CAD build for the part. Positions are in the model's coordinates, mm. A direction names the side the tool comes from. Round coordinates to 2 decimals unless told otherwise and drop trailing zeros. Order: outer loops, then holes, each group sorted by start corner. A loop starts at its lowest first (then second) coordinate and runs counter-clockwise, first axis right, second up. Notation, with made-up numbers: M 37.5,43 L 61.5,43 A27 ccw 61.5,80 Z; hole C 20,-39.5 d4. An arc over 180 degrees is marked long. Put each result on its own line as item: value.
Autodesk Inventor part; units mm, degrees
ref_plane "YZ Plane" through (0, 0, 0) normal (1, 0, 0) x (0, 1, 0)
ref_plane "XZ Plane" through (0, 0, 0) normal (0, 1, 0) x (-1, 0, 0)
ref_plane "XY Plane" through (0, 0, 0) normal (0, 0, 1) x (1, 0, 0)
sketch "草圖1" plane through (0, 0, 0) normal (0, 0, 1) x (1, 0, 0)
  line L0 (-27.5, 3) -> (27.5, 3) construction
  line L1 (27.5, 3) -> (27.5, 63) construction
  line L2 (27.5, 63) -> (-27.5, 63) construction
  line L3 (-27.5, 63) -> (-27.5, 3) construction
  line L4 (-30.5, 66) -> (30.5, 66)
  line L5 (30.5, 66) -> (30.5, -5.5597)
  line L6 (-30.5, -3) -> (-30.5, 66)
  line L7 (-34.7579, 0) -> (34.7579, 0)
  line L8 (-30.5, -66) -> (30.5, -66)
  line L9 (30.5, -66) -> (30.5, -5.5597)
  line L10 (-30.5, -3) -> (-30.5, -66)
  line L11 (0, 77.5612) -> (0, -87.4517)
  point P0 (0, 3)
  point P1 (0, 3)
  point P2 (0, -3)
  point P3 (0, 0)
  dimension "d0" = 55
  dimension "d1" = 60
  dimension "d2" = 3
  dimension "d3" = 6
extrude "擠出1" add sketch "草圖1" along normal blind 3 and the other way blind 70
shell "薄殼1" thickness 3 removed faces 1 at (-10.1667, 22, -70)
sketch "草圖2" plane through (0, 0, 0) normal (0, 0, 1) x (1, 0, 0)
  line L0 (27.5, 63) -> (27.5, -4)
  line L1 (27.5, -4) -> (-27.5, -4)
  line L2 (-27.5, -4) -> (-27.5, 63)
  line L3 (0, 77.5612) -> (0, -87.4517)
  line L4 (-34.7579, 0) -> (34.7579, 0)
  line L5 (27.5, 63) -> (-27.5, 63)
  point P0 (0, 0)
  point P1 (-27.5, 0)
  point P2 (27.5, 0)
  dimension "d8" = 55
  dimension "d9" = 8
extrude "擠出2" cut sketch "草圖2" along normal blind 3 and the other way blind 2
sketch "草圖3" plane through (0, 0, 0) normal (1, 0, 0) x (0, 1, 0)
  circle A0 centre (59, 0) radius 1.25
  line L0 (-66, 3) -> (66, 3)
  line L1 (-4, 0) -> (-4, 3) construction
  line L2 (2, 0) -> (2, 3) construction
  dimension "d13" = 2.5
  dimension "d17" = 3
  dimension "d20" = 6
  dimension "d21" = 57
extrude "擠出3" cut sketch "草圖3" along normal through all both and the other way through all
sketch "草圖4" plane through (0, 0, 0) normal (1, 0, 0) x (0, 1, 0)
  line L0 (66, -70) -> (-66, -70)
  line L1 (1.4687, -70) -> (0, -70)
  line L2 (77.5612, 0) -> (-87.4517, 0)
  line L3 (3, 1) -> (3, -70)
  line L4 (3, -70) -> (-1, -70)
  line L5 (-1, -70) -> (-1, 1)
  line L6 (-4, 0) -> (-4, 3)
  line L7 (3, 1) -> (-1, 1)
  point P0 (0, 0)
  point P1 (3, 0)
  point P2 (3, 0)
  point P3 (3, 0)
  dimension "d39" = 71
  dimension "d40" = 4
extrude "擠出4" add sketch "草圖4" along normal mid plane 55
sketch "草圖5" plane through (0, 0, 3) normal (0, 0, 1) x (1, 0, 0)
  line L0 (-30.5, 66) -> (-30.5, -66)
  line L1 (-30.5, -4) -> (30.5, -4)
  line L2 (30.5, -4) -> (30.5, 2.5)
  line L3 (-30.5, 2.5) -> (-30.5, -4)
  line L4 (27.5, -4) -> (-27.5, -4)
  line L5 (30.5, -66) -> (30.5, 66)
  circle A0 centre (-27.5, 0.7) radius 1.25 construction
  line L6 (-27.5, 3) -> (27.5, 3)
  line L7 (-27.5, 3) -> (27.5, 3)
  line L8 (27.5, 3) -> (27.5, 2.5)
  line L9 (-27.5, 2.5) -> (-27.5, 3)
  line L10 (-30.5, 2.5) -> (-27.5, 2.5)
  line L11 (27.5, 2.5) -> (30.5, 2.5)
  line L12 (27.5, 63) -> (27.5, -4) construction
  point P0 (0, 0)
  dimension "d41" = 2.5
  dimension "d42" = 3
  dimension "d46" = 6.5
extrude "擠出5" cut sketch "草圖5" against normal blind 3
sketch "草圖6" plane through (-27.5, -63, 0) normal (1, 0, 0) x (0, 0, -1)
  line L0 (0, 63) -> (3, 63)
  line L1 (3, 63) -> (3, 59)
  line L2 (3, 59) -> (0, 59)
  line L3 (0, 59) -> (0, 63)
  line L4 (-3, 59) -> (0, 59)
  dimension "d37" = 3
extrude "擠出6" add sketch "草圖6" along normal up to surface (55 mm away)
sketch "草圖7" plane through (-30.5, -4, 0) normal (0, 0, 1) x (1, 0, 0)
  circle A0 centre (3, 4.7) radius 1.5
  circle A1 centre (13, 1.5) radius 1.5
  line L0 (61, 0) -> (0, 0)
  line L1 (30.5, 81.5612) -> (30.5, -83.4517)
  circle A2 centre (58, 4.7) radius 1.5
  circle A3 centre (48, 1.5) radius 1.5
  line L2 (0, 0) -> (0, 6.5)
  line L3 (0, 6.5) -> (3, 6.5)
  point P0 (30.5, 4)
  point P1 (0, 4)
  point P2 (58, 0)
  dimension "d30" = 3
  dimension "d31" = 3
  dimension "d32" = 35
  dimension "d38" = 3
  dimension "d45" = 1.8
extrude "擠出7" cut sketch "草圖7" against normal blind 3
equation "\"d8\" = d0"
properties part number "frame"
Item 1: Band-saw the part on B-B on z = -15. Give the cut face in (x, y).
Answers below:
outline: M -30.5,-66 L 30.5,-66 L 30.5,66 L -30.5,66 Z; hole M -27.5,-63 L 27.5,-63 L 27.5,-1 L -27.5,-1 Z; hole M -27.5,3 L 27.5,3 L 27.5,63 L -27.5,63 Z
Item 2: Mould opens along X. For faces 1 (the flat face through (0, 65, 3)), 2 (the flat face through (-30.5, -1, -34)), 3 (the flat face through (0, -4, -2)) say: pulls with the +X half, pulls with the -X half, needs draft (parallel to the pull), parting line crosses it, or undercut.
Answers below:
face 1: needs draft
face 2: pulls with the -X half
face 3: undercut
Item 3: Band-saw the part on D-D on y = 54.5. Give the cut face in (x, z).
Answers below:
outline: M -30.5,-70 L -27.5,-70 L -27.5,3 L -30.5,3 Z; M 27.5,-70 L 30.5,-70 L 30.5,3 L 27.5,3 Z
Item 4: Pin check, flat tips, straight feed: P1, Ø3.5, axis at x = 5.5, y = 0, coming from the +Z side; P2, Ø6, axis at x = 1.5, y = -49, coming from the -Z side; P3, Ø2.5, axis at x = 27.5, y = 0.5, coming from the +Z side. Stop position of each tip, or through.
Answers below:
P1: z = 0
P2: z = 0
P3: z = -3
Item 5: Tool access for faces 4 (the flat face through (27, 1, -3)), 5 (the flat face through (0, -4, 2)), 6 (the flat face through (27.5, -32, -35)): list every direction of +Z, -Z, +X, -X, +Y, -Y with a clear straight run to the whole face (end or side of a thin tool).
Answers below:
face 4: +Z
face 5: +Z, +X, -X
face 6: -Z
Item 6: Band-saw the part on C-C on y = -28.5. Give the cut face in (x, z).
Answers below:
outline: M -30.5,-70 L -27.5,-70 L -27.5,0 L 27.5,0 L 27.5,-70 L 30.5,-70 L 30.5,3 L -30.5,3 Z
Item 7: Probe line 1 along X through (y, z) = (-2.5, -1.05); line 2 along Y through (x, z) = (23.5, -62); line 3 along X through (y, z) = (1, -2.5). List the from-to ranges inside material, lowest first. Write a range as [from, to].
Answers below:
line 1: [-30.5, -19], [-16, 16], [19, 30.5]
line 2: [-66, -63], [-1, 3], [63, 66]
line 3: [-30.5, -28.97], [-26.03, 26.03], [28.97, 30.5]
